Autodesk Inventor part; units mm, degrees
ref_plane "YZ Plane" through (0, 0, 0) normal (1, 0, 0) x (0, 1, 0)
ref_plane "XZ Plane" through (0, 0, 0) normal (0, 1, 0) x (-1, 0, 0)
ref_plane "XY Plane" through (0, 0, 0) normal (0, 0, 1) x (1, 0, 0)
sketch "스케치1" plane through (0, 0, 0) normal (1, 0, 0) x (0, 1, 0)
  line L0 (-12.35, 41) -> (12.35, 41)
  line L1 (12.35, 41) -> (12.35, -41)
  line L2 (12.35, -41) -> (-12.35, -41)
  line L3 (-12.35, -41) -> (-12.35, 41)
  line L4 (-12.35, 41) -> (12.35, -41) construction
  line L5 (12.35, 41) -> (-12.35, -41) construction
  point P0 (0, 0)
  dimension "d0" = 24.7
  dimension "d1" = 82
extrude "돌출1" add sketch "스케치1" along normal blind 82
ref_plane "작업 평면1" through (41, 0, 0) normal (1, 0, 0) x (0, 0, -1)
sketch "스케치2" plane through (41, 0, 0) normal (1, 0, 0) x (0, 0, -1)
  line L0 (-41, 12.35) -> (-41, -12.35)
  line L1 (-41, -12.35) -> (41, -12.35)
  line L2 (41, -12.35) -> (41, 12.35)
  line L3 (41, 12.35) -> (-41, 12.35)
  line L4 (0, -12.35) -> (0, -62.35)
  circle A0 centre (0, -62.35) radius 37.5
  point P0 (0, 0)
  dimension "d5" = 50
  dimension "d6" = 75
extrude "돌출2" add sketch "스케치2" along normal mid plane 32 contours A0
sketch "스케치3" plane through (57, -62.35, 0) normal (1, 0, 0) x (0, 0, -1)
  line L0 (-41, 50) -> (41, 50)
  line L1 (0, 50) -> (-15, 50)
  line L2 (-15, 50) -> (-15, 0)
  line L3 (-15, 0) -> (15, 0)
  line L4 (15, 0) -> (15, 50)
  point P0 (0, 62.35)
  dimension "d9" = 15
  dimension "d10" = 50
  dimension "d11" = 30
extrude "돌출3" add sketch "스케치3" along normal blind 4
sketch "스케치4" plane through (25, -62.35, 0) normal (-1, 0, 0) x (0, 0, 1)
  line L0 (0, 0) -> (-15, 0)
  line L1 (-15, 0) -> (-15, 50)
  line L2 (41, 50) -> (-41, 50)
  line L3 (15, 50) -> (15, 34.3693)
  line L4 (15, 50) -> (15, 0)
  line L5 (15, 0) -> (15, 34.3693)
  line L6 (-15, 0) -> (15, 0)
  line L7 (15, 50) -> (-15, 50)
  point P0 (0, 62.35)
extrude "돌출4" add sketch "스케치4" along normal blind 4
properties part number "Caster" material "고무"
Input: part model. Units: mm. Frame: model coordinates. A direction names the side the tool comes from. Give positions to 0.01 mm unless a question says otherwise; leave off trailing zeros. Order: outer loops, then holes, each group sorted by start corner. A loop starts at its lowest first (then second) coordinate and runs counter-clockwise, first axis right, second up. Notation, with made-up numbers: (78.25, 8) -> (99.25, 8) arc R21 cw to (99.25, 16) -> close; hole circle Ø4 at (75, 67.25). An arc over 180 degrees is marked (long way). Write each question's results on one line, items separated by ' | '. Start each with the question number.
Item 1: Cut plane D-D on x = 10. Return the cut outline in (y, z), then the cut area to 3 significant figures.
Item 2: Set-up query: faces 4 (the flat face through (59, -38, -15)), 5 (the flat face through (59, -62.35, 0)), 6 (the flat face through (23, -37, 15)), 7 (the flat face through (23, -62.35, 0)). Return all of +Z, -Z, +X, -X, +Y, -Y with unobstructed straight access to the full face (end or side cutting, diameter ignored); none if empty.
Item 3: Mould query, pull axis X, two halves, no side actions, for faces 1 (the flat face through (21, -37, 0)), 2 (the flat face through (25, -18, 0)), 3 (the flat face through (59, -37, 15)). Classes: pulls with the +X half, pulls with the -X half, needs draft (parallel to the pull), parting line crosses it, or undercut.
Item 4: Line query: line 1 (X direction, y = -24.5, z = 7); line 2 (Y direction, x = 15, z = 15.5); line 3 (Z direction, x = 60, y = -55). Output: solid intervals per line, ascending.
Item 5: Cut plane B-B on x = 51.5. Return the cut outline in (y, z).
Item 6: Cut plane C-C on z = 0. Return the cut outline in (x, y).
Item 7: Contact query for flat-ended pins moving along their axis: P1, Ø2, axis at x = 23, y = -41.5, coming from the -Z side; P2, Ø9, axis at y = -28, z = 3.5, coming from the -X side; P3, Ø1, axis at y = -74, z = 8.5, coming from the -X side. Output: stop coordinate, or through.
Item 8: Cut plane A-A on y = -16. Return the cut outline in (x, z).
Established:
1) outline: (-12.35, -41) -> (12.35, -41) -> (12.35, 41) -> (-12.35, 41) -> close | area: 2,030 mm^2
2) face 4: -Z, +X, -Y | face 5: +Z, -Z, +X, -Y | face 6: +Z, -X, -Y | face 7: +Z, -Z, -X, -Y
3) face 1: pulls with the -X half | face 2: undercut | face 3: needs draft
4) line 1: 21 to 25, 57 to 61 | line 2: -12.35 to 12.35 | line 3: -15 to 15
5) outline: circle Ø75 at (-62.35, 0); (-12.35, -41) -> (12.35, -41) -> (12.35, 41) -> (-12.35, 41) -> close
6) outline: (0, -12.35) -> (21, -12.35) -> (21, -62.35) -> (25, -62.35) -> (25, -99.85) -> (57, -99.85) -> (57, -62.35) -> (61, -62.35) -> (61, -12.35) -> (82, -12.35) -> (82, 12.35) -> (0, 12.35) -> close; hole (25, -24.85) -> (57, -24.85) -> (57, -12.35) -> (25, -12.35) -> close
7) P1: z = -15 | P2: x = 21 | P3: x = 25
8) outline: (21, -15) -> (25, -15) -> (25, 15) -> (21, 15) -> close; (57, -15) -> (61, -15) -> (61, 15) -> (57, 15) -> close
